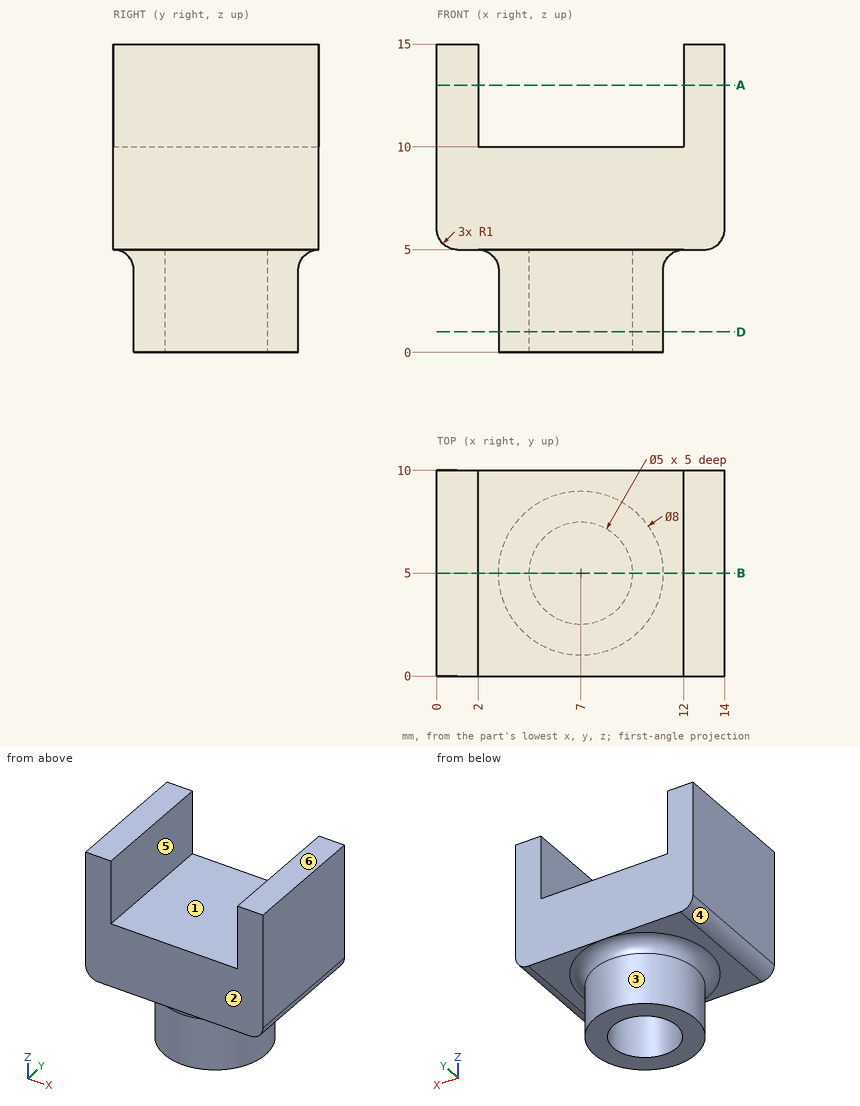
Geometry: see drawing. Coordinates: mm, zero at the bounding-box minimum. A direction names the side the tool comes from. Give positions to 0.01 mm unless a question says otherwise; leave off trailing zeros. Loops run counter-clockwise (first coordinate to the right, second up) from the corner with the lowest first, then second, coordinate; pieces in that order, holes last. Notation, with made-up numbers: (-1, 4.5) - (20, 4.5) arc R26 cw to (20, 33.5) - close; hole circle Ø8 at (72, 80). An arc over 180 degrees is marked (long way). Use CSV: the item, a comma, the result in double quotes. Start each with the question number.
Item 1: Section A-A on z = 13. Return loops of the section in (x, y), then the cut area to 3 significant figures.
Item 2: Section D-D on z = 1. Return loops of the section in (x, y).
Item 3: Line query: line 1 (Y direction, x = 7, z = 2.6); line 2 (X direction, y = 3.25, z = 10.75); line 3 (Z direction, x = 5.25, y = 6.75). Output: solid intervals per line, ascending.
Item 4: Reachability of the marked faces 1, 2 and 3 from +Z, -Z, +X, -X, +Y, -Y: full face, straight path, thin tool, end or side. Return the list, or none.
Item 5: Section B-B on y = 5. Return loops of the section in (x, z), then the cut area to 3 significant figures.
Item 6: Mould query, pull axis X, two halves, no side actions, for the marked faces 4, 5 and 6. Classes: pulls with the +X half, pulls with the -X half, needs draft (parallel to the pull), parting line crosses it, or undercut.
Item 7: Contact query for flat-ended pins moving along their axis: P1, Ø1.5, axis at x = 6.5, y = 5.5, coming from the -Z side; P2, Ø5, axis at x = 10.5, z = 5, coming from the -Y side. Output: stop coordinate, or through.
Ans:
1,outline,"(0, 0) - (2, 0) - (2, 10) - (0, 10) - close; (12, 0) - (14, 0) - (14, 10) - (12, 10) - close"
1,area,"40.0 mm2"
2,outline,"circle Ø8 at (7, 5); hole circle Ø5 at (7, 5)"
3,line 1,"y = 1 to 2.5, 7.5 to 9"
3,line 2,"x = 0 to 2, 12 to 14"
3,line 3,"z = 5 to 10"
4,face 1,"+Z, +Y, -Y"
4,face 2,"+Z, -Z, +X, -X, -Y"
4,face 3,"-Z"
5,outline,"(0, 6) arc R1 ccw to (1, 5) - (2, 5) arc R1 cw to (3, 4) - (3, 0) - (4.5, 0) - (4.5, 5) - (9.5, 5) - (9.5, 0) - (11, 0) - (11, 4) arc R1 cw to (12, 5) - (13, 5) arc R1 ccw to (14, 6) - (14, 15) - (12, 15) - (12, 10) - (2, 10) - (2, 15) - (0, 15) - close"
5,area,"105 mm2"
6,face 4,"pulls with the -X half"
6,face 5,"undercut"
6,face 6,"needs draft"
7,P1,"stops at z = 5"
7,P2,"stops at y = 0"
